The listing builds one solid part. Answer for the finished solid, in the listing's coordinates (mm). A direction names the side the tool comes from. Round coordinates to 2 decimals unless told otherwise and drop trailing zeros. Loops run counter-clockwise (first coordinate to the right, second up) from the corner with the lowest first, then second, coordinate; pieces in that order, holes last. Notation, with made-up numbers: (68.25, -39) -> (110.25, -39) arc R20 cw to (110.25, -19) -> close; hole circle Ø5 at (-23, -20.75). An arc over 180 degrees is marked (long way). Write each question's results on one line, items separated by ' | '. Start each with the question number.
(1) The part is cut by section D-D (z = 9.5). Determine the outline of the cut face in (x, y).
(2) For faces 1 (the face through (-347.133, 2, 7)), 2 (the face through (-348.933, 2, 7)), 3 (the face through (-342, 2.6, 6)), 4 (the face through (-348, 2, 5.018)), determine the directions among +Z, -Z, +X, -X, +Y, -Y from which every point of the face is accessible in a straight line to the end or side of a thin tool.
(3) Straight lines are drawn through the part: probe 1 along Z at (x, y) = (-341.25, 2.2); probe 2 along Y at (x, z) = (-344.25, 2); probe 3 along X at (y, z) = (2.1, 4.5). For each, find the intervals that lie inside material, in ascending order.
(4) Flat-ended cylindrical pins translate along their axes: pin 1 (1.2 mm diameter, centred on x = -348, y = 2, fed in from +Z); pin 2 (1.7 mm diameter, centred on x = -343, z = 6.5, fed in from +Y); pin 3 (0.9 mm diameter, centred on y = 2.5, z = 6, fed in from -X). Find the tip coordinate at first contact, or state that the pin passes through.
(5) The part is cut by section B-B (z = 4.5). Determine the outline of the cut face in (x, y), plus the area to 3 significant figures.
(6) The part is cut by section C-C (x = -342.5). Determine the outline of the cut face in (y, z), plus the area to 3 significant figures.
(7) Determine the mould class of faces 5 (the face through (-348, 2, 8.018)), 6 (the face through (-346, 1.6, 7)), 7 (the face through (-353.056, 0.811, 6.558)) for opening direction Z: released by +Z, released by -Z, zero draft, split by the parting line, or undercut.
(8) The part is cut by section A-A (x = -347.75). Determine the outline of the cut face in (y, z), plus the area to 3 significant figures.
```python
from build123d import *

# Parameters (mm, degrees)
SKETCH1_W        = 14.75
SKETCH1_H        = 10.85
MIC_BOARD_DEPTH  = 1.6
SKETCH2_R        = 0.5
PINS_DEPTH       = 1.6
MIC_SKETCH_W     = 4
MIC_SKETCH_H     = 4.2
MICROPHONE_DEPTH = 1
OP_AMP_SKETCH_W  = 1.8
OP_AMP_SKETCH_H  = 3
OP_AMP_DEPTH     = 1.2
MIC_FILLET_R     = 0.3
OP_AMP_FILLET_R  = 0.1


with BuildPart() as part:
    # Sketch1 → Mic Board (new body)
    with BuildSketch(Plane(origin=(0, 0, 0), x_dir=(1, 0, 0), z_dir=(0, 1, 0))):
        with Locations((-347.05792854, -6.593292201)):
            Rectangle(SKETCH1_W, SKETCH1_H)
    extrude(amount=MIC_BOARD_DEPTH)

    # Sketch2 → Pins (cut)
    with BuildSketch(Plane(origin=(0, 1.6, 0), x_dir=(1, 0, 0), z_dir=(0, 1, 0))):
        with Locations((-353.53292854, -4.168292201)):
            Circle(SKETCH2_R)
        with Locations((-353.53292854, -6.708292201)):
            Circle(SKETCH2_R)
        with Locations((-353.53292854, -9.248292201)):
            Circle(SKETCH2_R)
    extrude(amount=-PINS_DEPTH, mode=Mode.SUBTRACT)

    # mic Sketch → Microphone (add)
    with BuildSketch(Plane(origin=(0, 1.6, 0), x_dir=(1, 0, 0), z_dir=(0, 1, 0))):
        with Locations((-342.33292854, -6.118292201)):
            Rectangle(MIC_SKETCH_W, MIC_SKETCH_H)
    extrude(amount=MICROPHONE_DEPTH)

    # Op Amp Sketch → Op Amp (add)
    with BuildSketch(Plane(origin=(0, 1.6, 0), x_dir=(1, 0, 0), z_dir=(0, 1, 0))):
        with Locations((-348.03292854, -6.518292201)):
            Rectangle(OP_AMP_SKETCH_W, OP_AMP_SKETCH_H)
    extrude(amount=OP_AMP_DEPTH)

    # Mic Fillet
    mic_fillet_edges = [part.edges().sort_by_distance(p)[0] for p in [
        (-342.33292854, 2.6, 4.018292201),
        (-344.33292854, 1.6, 6.118292201),
        (-342.33292854, 1.6, 8.218292201),
        (-340.33292854, 2.6, 6.118292201),
        (-344.33292854, 2.6, 6.118292201),
        (-342.33292854, 2.6, 8.218292201),
        (-342.33292854, 1.6, 4.018292201),
        (-340.33292854, 1.6, 6.118292201),
    ]]
    fillet(mic_fillet_edges, radius=MIC_FILLET_R)

    # Op Amp Fillet
    op_amp_fillet_edges = [part.edges().sort_by_distance(p)[0] for p in [
        (-348.93292854, 2.8, 6.518292201),
        (-348.03292854, 2.8, 8.018292201),
        (-347.13292854, 2.8, 6.518292201),
        (-348.03292854, 2.8, 5.018292201),
    ]]
    fillet(op_amp_fillet_edges, radius=OP_AMP_FILLET_R)


solid = part.part
```
Checked values:
1) outline: (-354.43, 0) -> (-353.96, 0) -> (-353.96, 1.6) -> (-354.43, 1.6) -> close; (-353.1, 0) -> (-339.68, 0) -> (-339.68, 1.6) -> (-353.1, 1.6) -> close
2) face 1: +Z, -Z, +Y | face 2: +Z, -Z, -X, +Y | face 3: +Z, -Z, +X, +Y | face 4: -Z, -X, +Y
3) probe 1: z = 4.02 to 8.22 | probe 2: y = 0 to 1.6 | probe 3: x = -344.33 to -340.33
4) pin 1: stops at z = 12.02 | pin 2: stops at y = 2.6 | pin 3: stops at x = -348.93
5) outline: (-354.43, 0) -> (-353.91, 0) -> (-353.91, 1.6) -> (-354.43, 1.6) -> close; (-353.16, 0) -> (-339.68, 0) -> (-339.68, 1.6) -> (-340.03, 1.6) arc R0.3 cw to (-340.33, 1.9) -> (-340.33, 2.3) arc R0.3 ccw to (-340.63, 2.6) -> (-344.03, 2.6) arc R0.3 ccw to (-344.33, 2.3) -> (-344.33, 1.9) arc R0.3 cw to (-344.63, 1.6) -> (-353.16, 1.6) -> close | area: 26.4 mm2
6) outline: (0, 1.17) -> (1.6, 1.17) -> (1.6, 3.72) arc R0.3 cw to (1.9, 4.02) -> (2.3, 4.02) arc R0.3 ccw to (2.6, 4.32) -> (2.6, 7.92) arc R0.3 ccw to (2.3, 8.22) -> (1.9, 8.22) arc R0.3 cw to (1.6, 8.52) -> (1.6, 12.02) -> (0, 12.02) -> close | area: 21.6 mm2
7) face 5: released by +Z | face 6: zero draft | face 7: undercut
8) outline: (0, 1.17) -> (1.6, 1.17) -> (1.6, 5.02) -> (2.7, 5.02) arc R0.1 ccw to (2.8, 5.12) -> (2.8, 7.92) arc R0.1 ccw to (2.7, 8.02) -> (1.6, 8.02) -> (1.6, 12.02) -> (0, 12.02) -> close | area: 21.0 mm2
